```python
from build123d import *

# Parameters (mm, degrees)
FILLET_1_R          = 0.16
SKETCH_2_R          = 2
EXTRUDE_1_DEPTH     = 20
FILLET_2_R          = 0.16
CUT_EXTRUDE_1_DEPTH = 1


with BuildPart() as part:
    # 草图1 → 旋转1 (revolve)
    with BuildSketch(Plane.XY):
        Polygon((0, 0), (0, 3.5), (2.5, 2), (2.5, 0), align=None)
    revolve(axis=Axis((0, 0, 0), (-1, 0, 0)))

    # 圆角1
    fillet_1_edges = [part.edges().sort_by_distance(p)[0] for p in [
        (0, -3.5, 0),
    ]]
    fillet(fillet_1_edges, radius=FILLET_1_R)

    # 草图2 → 凸台-拉伸1 (add)
    with BuildSketch(Plane(origin=(2.5, 0, 0), x_dir=(0, 0, -1), z_dir=(1, 0, 0))):
        Circle(SKETCH_2_R)
    extrude(amount=EXTRUDE_1_DEPTH)

    # 圆角2
    fillet_2_edges = [part.edges().sort_by_distance(p)[0] for p in [
        (22.5, 0, 2),
    ]]
    fillet(fillet_2_edges, radius=FILLET_2_R)

    # 草图3 → 切除-拉伸1 (cut)
    with BuildSketch(Plane.ZY):
        Polygon((0.41, -0.41), (0.41, -2.15), (-0.41, -2.15), (-0.41, -0.41), (-2.15, -0.41), (-2.15, 0.41), (-0.41, 0.41), (-0.41, 2.15), (0.41, 2.15), (0.41, 0.41), (2.15, 0.41), (2.15, -0.41), align=None)
    extrude(amount=-CUT_EXTRUDE_1_DEPTH, mode=Mode.SUBTRACT)


solid = part.part
```
The listing builds one solid part. Answer for the finished solid, in the listing's coordinates (mm). A direction names the side the tool comes from. Give positions to 0.01 mm unless a question says otherwise; leave off trailing zeros. Loops run counter-clockwise (first coordinate to the right, second up) from the corner with the lowest first, then second, coordinate; pieces in that order, holes last. Notation, with made-up numbers: (25.5, 38.5) - (49.5, 38.5) arc R38 ccw to (49.5, 77.5) - close; hole circle Ø6 at (-13, -36.5). An arc over 180 degrees is marked (long way). Answer as CSV lines item,"result". Start each with the question number.
Item 1: A cutting plane is placed at C-C on x = 19. Determine the outline of the cut face in (y, z), then the cut area to 3 significant figures.
Item 2: For faces 1 (the face through (0.5, -1.3, 0.41)), 2 (the face through (0, -1, 1)), determine the directions among +Z, -Z, +X, -X, +Y, -Y from which every point of the face is accessible in a straight line to the end or side of a thin tool.
Item 3: A cutting plane is placed at A-A on y = 0. Determine the outline of the cut face in (x, z), then the cut area to 3 significant figures.
Item 4: Find the intervals of material crossed by line 1 (X direction, y = -0.75, z = -0.25); line 2 (Y direction, x = 10.5, z = -0.25); line 3 (X direction, y = 0.5, z = 2.25), in increasing order. Write a range as from..to.
Item 5: The mould has two halves that part along Z. Classify faces 3 (the face through (22.5, 0, 0)), 4 (the face through (0.5, -0.41, 1.3)), 5 (the face through (12, -2, 0)): +Z half, -Z half, draft (parallel to the pull), parting line (faces both ways), or undercut.
Item 6: Each of these flat-tipped pins is pushed along its axis until it touches: pin 1 (0.8 mm diameter, centred on x = 0.5, z = 1, fed in from -Y); pin 2 (1.5 mm diameter, centred on x = 8, z = 2.5, fed in from -Y); pin 3 (0.5 mm diameter, centred on x = 0.5, y = -1.5, fed in from -Z). Where does it stop, or does it pass through?
Found:
1,outline,"circle Ø4 at (0, 0)"
1,area,"12.6 mm^2"
2,face 1,"-X"
2,face 2,"+Z, -Z, -X, +Y, -Y"
3,outline,"(0, -3.22) arc R0.16 ccw to (0.24, -3.35) - (2.5, -2) - (22.34, -2) arc R0.16 ccw to (22.5, -1.84) - (22.5, 1.84) arc R0.16 ccw to (22.34, 2) - (2.5, 2) - (0.24, 3.35) arc R0.16 ccw to (0, 3.22) - (0, 2.15) - (1, 2.15) - (1, -2.15) - (0, -2.15) - close"
3,area,"89.4 mm^2"
4,line 1,"x = 1..22.5"
4,line 2,"y = -1.98..1.98"
4,line 3,"x = 0..1.99"
5,face 3,"draft"
5,face 4,"undercut"
5,face 5,"parting line"
6,pin 1,"stops at y = -3.29"
6,pin 2,"stops at y = -0.97"
6,pin 3,"stops at z = -3.03"
